Work out the finished part from the listing and answer in its coordinate system (mm). A direction names the side the tool comes from. Give positions to 0.01 mm unless a question says otherwise; leave off trailing zeros. Write each loop counter-clockwise with the first axis right and the second up, starting at its lowest first coordinate (ties: lowest second). Pieces come first, ordered by that corner, then holes. Notation, with made-up numbers: (-11.5, 42) -> (13.5, 42) arc R13 ccw to (13.5, 62) -> close; hole circle Ø7 at (4, 30.5). An arc over 180 degrees is marked (long way). Write item = value, one per line. Start each with the question number.
from build123d import *

# Parameters (mm, degrees)
SKETCH2_R           = 30.1625
SKETCH2_R_2         = 26.2509
BOSS_EXTRUDE1_START = -9.525
SKETCH9_R           = 34.9377
SKETCH9_R_2         = 30.1625
BOSS_EXTRUDE1_DEPTH = 28.575
CHAMFER1_SIZE       = 10


with BuildPart() as part:
    # Sweep2: sweep along a path in Sketch1
    with BuildLine(Plane(origin=(0, 0, 0), x_dir=(0, 0, -1), z_dir=(1, 0, 0))) as sweep2_path:
        Line((-63.5, 0), (-38.1, 0))
        ThreePointArc((-38.1, 0), (-11.159231637, -11.159231637), (0, -38.1))
        Line((0, -38.1), (0, -63.5))
    # Sketch2 → Sweep2 (sweep)
    with BuildSketch(Plane.XY.offset(63.5)):
        Circle(SKETCH2_R)
        Circle(SKETCH2_R_2, mode=Mode.SUBTRACT)
    sweep(path=sweep2_path.line)

    # Sketch9 → Boss-Extrude1 (add)
    with BuildSketch(Plane.XY.offset(63.5).offset(BOSS_EXTRUDE1_START)):
        with Locations(Location((0, 0, 0), (0, 0, 180))):
            Circle(SKETCH9_R)
        Circle(SKETCH9_R_2, mode=Mode.SUBTRACT)
    boss_extrude1 = extrude(amount=BOSS_EXTRUDE1_DEPTH)

    # Mirror4: Boss-Extrude1 across plane
    add(boss_extrude1.mirror(Plane(origin=(0, 0, 0), x_dir=(0, -0.7071067811865465, 0.7071067811865486), z_dir=(0, 0.7071067811865488, 0.7071067811865464))))

    # Chamfer1
    # the kernel refuses this chamfer: 10 mm, written as the material it adds along each edge
    with BuildSketch(Plane(origin=(0, 0, 53.975), x_dir=(1, 0, 0), z_dir=(0, -1, 0))) as chamfer1_piece_1_section:
        Polygon((30.1625, -CHAMFER1_SIZE), (30.1625 + CHAMFER1_SIZE, 0), (30.1625, 0), align=None)
    chamfer1_piece_1 = revolve(axis=Axis((0, 0, 53.975), (0, 0, 1)), mode=Mode.PRIVATE)
    chamfer1_piece_1 = chamfer1_piece_1 & Plane(origin=(0, 0, 46.362739963), x_dir=(-1, 0, 0), z_dir=(0, 0, -1)) * Cylinder(34.9377, 161, mode=Mode.PRIVATE)
    add(chamfer1_piece_1)
    with BuildSketch(Plane(origin=(0, -53.975, 0), x_dir=(1, 0, 0), z_dir=(0, 0, 1))) as chamfer1_piece_2_section:
        Polygon((30.1625, CHAMFER1_SIZE), (30.1625 + CHAMFER1_SIZE, 0), (30.1625, 0), align=None)
    chamfer1_piece_2 = revolve(axis=Axis((0, -53.975, 0), (0, 1, 0)), mode=Mode.PRIVATE)
    chamfer1_piece_2 = chamfer1_piece_2 & Plane(origin=(0, -46.362739963, 0), x_dir=(-1, 0, 0), z_dir=(0, 1, 0)) * Cylinder(34.9377, 161, mode=Mode.PRIVATE)
    add(chamfer1_piece_2)


solid = part.part
(1) Determine the mould class of faces 1 (the cylindrical face through (4.55, 34.64, 65.41)), 2 (the cylindrical face through (-30.133, 1.326, 72.892)), 3 (the flat face through (29, 10, 82.55)) for opening direction X: pulls with the +X half, pulls with the -X half, needs draft (parallel to the pull), parting line crosses it, or undercut.
(2) Each of these flat-tipped pins is pushed along its axis until it touches: pin 1 (10 mm diameter, centred on x = 9.5, y = -23, fed in from -Z); pin 2 (3 mm diameter, centred on x = 10.5, y = -65.5, fed in from +Z); pin 3 (1 mm diameter, centred on x = -2, y = 18.5, fed in from +Z). Where does it stop, or does it pass through?
(3) A cutting plane is placed at B-B, the plane z = 57. Write down the section's boundary in (x, y).
(4) A cutting plane is placed at C-C, the plane y = -71.5. Write down the section's boundary in (x, z) (1 decimal).
(5) For faces 4 (the cylindrical face through (-3.417, -26.028, 50.622)), 5 (the flat face through (29, -82.55, -10)), 6 (the cylindrical face through (-30.133, -41.079, 1.326)), 7 (the cylindrical face through (4.55, -65.41, 34.64)), determine the directions among +Z, -Z, +X, -X, +Y, -Y from which every point of the face is accessible in a straight line to the end or side of a thin tool.
(6) Find the intervals of material crossed by line 1 along Z through (x, y) = (0, -43.75); line 2 along X through (y, z) = (0, 75.25), in increasing order.
Results list:
q1.face_1 = parting line crosses it
q1.face_2 = undercut
q1.face_3 = needs draft
q2.pin_1 = -28.57
q2.pin_2 = 33.76
q2.pin_3 = 8.59
q3.outline = circle Ø69.88 at (0, 0); hole circle Ø52.5 at (0, 0)
q4.outline = circle Ø69.9 at (0, 0); hole circle Ø60.3 at (0, 0)
q5.face_4 = +Z
q5.face_5 = +Z, -Z, +X, -X, -Y
q5.face_6 = none
q5.face_7 = -Y
q6.line_1 = -30.16 to -26.25, 26.25 to 30.16
q6.line_2 = -34.94 to -30.16, 30.16 to 34.94
